Part model, mm, in its own coordinate system. Face numbers are marked on the shaded views. A direction names the side the tool comes from. Round coordinates to 2 decimals unless told otherwise and drop trailing zeros. Loops run counter-clockwise (first coordinate to the right, second up) from the corner with the lowest first, then second, coordinate; pieces in that order, holes last. Notation, with made-up numbers: (45, -30) - (90, -30) arc R17 cw to (90, -9) - close; hole circle Ø9 at (89.25, 32.25). An arc over 180 degrees is marked (long way). Write each question's results on one line, items separated by ' | '. Start each with the question number.
(1) Tool access for the marked faces 1, 2, 3, 4 and 5: list every direction of +Z, -Z, +X, -X, +Y, -Y with a clear straight run to the whole face (end or side of a thin tool).
(2) Cut at C-C, the plane y = 8. List the corners of the cut face in (x, z).
(3) Drill centre lines: L1, parallel to Z at x = 5.5, y = 2.2; L2, parallel to Z at x = 54.5, y = 22; L3, parallel to X at y = 1.45, z = -40.5. Where is each one in solid material? Low to high.
(4) Cut at A-A, the plane y = 29.5. List the corners of the cut face in (x, z), then the cut area to 3 significant figures.
(5) Flat gauge pins, fed straight in: P1, Ø11, axis at x = 53.5, z = -13, coming from the -Y side; P2, Ø8, axis at x = 35.5, y = 7.5, coming from the +Z side; P3, Ø5.5, axis at x = 52.5, z = -29.5, coming from the +Y side. Where does each tip first touch, or does it go through?
(6) Cut at B-B, the plane y = 17. List the corners of the cut face in (x, z), then the cut area to 3 significant figures.
(7) Cut at D-D, the plane z = 5. List the corners of the cut face in (x, y).
(8) Mould opens along Z. For the marked faces 6, 7, 8 and 9 say: released by +Z, released by -Z, zero draft, split by the parting line, or undercut.
from build123d import *

# Parameters (mm, degrees)
BOSS_EXTRUDE1_DEPTH = 3.8
SKETCH2_W           = 45.8
SKETCH2_H           = 50
BOSS_EXTRUDE2_DEPTH = 4
BOSS_EXTRUDE3_DEPTH = 46.2
BOSS_EXTRUDE4_DEPTH = 3.8
BOSS_EXTRUDE5_REACH = 52
SKETCH6_W           = 9
SKETCH6_H           = 50
BOSS_EXTRUDE6_DEPTH = 1
BOSS_EXTRUDE6_TAPER = 45
SKETCH7_R           = 2.6
BOSS_EXTRUDE7_DEPTH = 4
CUT_EXTRUDE1_REACH  = 6
SKETCH8_R           = 13
SKETCH8_R_2         = 1.6
SKETCH9_R           = 2.6
CUT_EXTRUDE2_DEPTH  = 4.8
SKETCH10_R          = 5
CUT_EXTRUDE3_DEPTH  = 20


with BuildPart() as part:
    # Sketch1 → Boss-Extrude1 (new body)
    with BuildSketch(Plane.XY):
        Polygon((0, 0), (45.8, 0), (64.164, 21.885362974), (64.164, 24.164), (44.164, 24.164), (44.164, 44.164), (40.164, 44.164), (0, 4), align=None)
    extrude(amount=-BOSS_EXTRUDE1_DEPTH)

    # Sketch2 → Boss-Extrude2 (add)
    with BuildSketch(Plane.XZ):
        with Locations((22.9, -25)):
            Rectangle(SKETCH2_W, SKETCH2_H)
    extrude(amount=-BOSS_EXTRUDE2_DEPTH)

    # Sketch3 → Boss-Extrude3 (add, through all)
    with BuildSketch(Plane(origin=(0, 0, -3.8), x_dir=(-1, 0, 0), z_dir=(0, 0, -1))):
        Polygon((-45.8, 0), (-45.8, 4), (-49.156398525, 4), align=None)
    extrude(amount=BOSS_EXTRUDE3_DEPTH)

    # Sketch4 → Boss-Extrude4 (add)
    with BuildSketch(Plane(origin=(0, 0, -50), x_dir=(-1, 0, 0), z_dir=(0, 0, -1))):
        Polygon((-44.164, 24.164), (-44.164, 44.164), (-40.164, 44.164), (0, 4), (0, 0), (-45.8, 0), (-64.164, 21.885362974), (-64.164, 24.164), align=None)
    extrude(amount=-BOSS_EXTRUDE4_DEPTH)

    # Sketch5 → Boss-Extrude5 (add, up to next)
    with BuildSketch(Plane.XY, mode=Mode.PRIVATE) as boss_extrude5_sk1:
        Polygon((44.164, 24.164), (44.164, 0), (45.8, 0), (64.164, 21.885362974), (64.164, 24.164), align=None)
    boss_extrude5_tool1 = extrude(boss_extrude5_sk1.sketch, amount=-BOSS_EXTRUDE5_REACH, mode=Mode.PRIVATE) - part.part
    add(boss_extrude5_tool1.solids().sort_by_distance((51.403304, 15.489129, 0))[0])

    # Sketch6 → Boss-Extrude6 (add)
    with BuildSketch(Plane(origin=(0, 24.164, 0), x_dir=(1, 0, 0), z_dir=(0, 1, 0))):
        with Locations((54.164, 25)):
            Rectangle(SKETCH6_W, SKETCH6_H)
    extrude(amount=BOSS_EXTRUDE6_DEPTH, taper=BOSS_EXTRUDE6_TAPER)

    # Sketch7 → Boss-Extrude7 (add)
    with BuildSketch(Plane(origin=(44.164, 0, 0), x_dir=(0, 0, -1), z_dir=(1, 0, 0))):
        with BuildLine():
            Line((0, 24.164), (0, 10.164))
            Line((0, 10.164), (-16.646029173, 27.168696786))
            ThreePointArc((-16.646029173, 27.168696786), (-18.718270774, 38.040013923), (-9.5, 44.164))
            Line((-9.5, 44.164), (3.8, 44.164))
            Line((3.8, 44.164), (3.8, 24.164))
            Line((3.8, 24.164), (0, 24.164))
        make_face()
        with Locations((-9.5, 34.164)):
            Circle(SKETCH7_R, mode=Mode.SUBTRACT)
        with BuildLine():
            Line((46.2, 44.164), (46.2, 24.164))
            Line((46.2, 24.164), (50, 24.164))
            Line((50, 24.164), (50, 10.164))
            Line((50, 10.164), (66.646029173, 27.168696786))
            ThreePointArc((66.646029173, 27.168696786), (68.718270774, 38.040013923), (59.5, 44.164))
            Line((59.5, 44.164), (46.2, 44.164))
        make_face()
        with Locations((59.5, 34.164)):
            Circle(SKETCH7_R, mode=Mode.SUBTRACT)
    extrude(amount=-BOSS_EXTRUDE7_DEPTH)

    # Sketch8 → Cut-Extrude1 (cut, up to next)
    with BuildSketch(Plane(origin=(0, 4, 0), x_dir=(1, 0, 0), z_dir=(0, 1, 0)), mode=Mode.PRIVATE) as cut_extrude1_sk1:
        with Locations((21, 25)):
            Circle(SKETCH8_R)
    cut_extrude1_tool1 = extrude(cut_extrude1_sk1.sketch, amount=-CUT_EXTRUDE1_REACH, mode=Mode.PRIVATE) & part.part
    add(cut_extrude1_tool1.solids().sort_by_distance((21, 4, -25))[0], mode=Mode.SUBTRACT)
    # Sketch8 → Cut-Extrude1 (cut, up to next)
    with BuildSketch(Plane(origin=(0, 4, 0), x_dir=(1, 0, 0), z_dir=(0, 1, 0)), mode=Mode.PRIVATE) as cut_extrude1_sk2:
        with Locations((5.5, 40.5)):
            Circle(SKETCH8_R_2)
    cut_extrude1_tool2 = extrude(cut_extrude1_sk2.sketch, amount=-CUT_EXTRUDE1_REACH, mode=Mode.PRIVATE) & part.part
    add(cut_extrude1_tool2.solids().sort_by_distance((5.5, 4, -40.5))[0], mode=Mode.SUBTRACT)
    # Sketch8 → Cut-Extrude1 (cut, up to next)
    with BuildSketch(Plane(origin=(0, 4, 0), x_dir=(1, 0, 0), z_dir=(0, 1, 0)), mode=Mode.PRIVATE) as cut_extrude1_sk3:
        with Locations((38.664, 40.5)):
            Circle(SKETCH8_R_2)
    cut_extrude1_tool3 = extrude(cut_extrude1_sk3.sketch, amount=-CUT_EXTRUDE1_REACH, mode=Mode.PRIVATE) & part.part
    add(cut_extrude1_tool3.solids().sort_by_distance((38.664, 4, -40.5))[0], mode=Mode.SUBTRACT)
    # Sketch8 → Cut-Extrude1 (cut, up to next)
    with BuildSketch(Plane(origin=(0, 4, 0), x_dir=(1, 0, 0), z_dir=(0, 1, 0)), mode=Mode.PRIVATE) as cut_extrude1_sk4:
        with Locations((38.664, 7.336)):
            Circle(SKETCH8_R_2)
    cut_extrude1_tool4 = extrude(cut_extrude1_sk4.sketch, amount=-CUT_EXTRUDE1_REACH, mode=Mode.PRIVATE) & part.part
    add(cut_extrude1_tool4.solids().sort_by_distance((38.664, 4, -7.336))[0], mode=Mode.SUBTRACT)
    # Sketch8 → Cut-Extrude1 (cut, up to next)
    with BuildSketch(Plane(origin=(0, 4, 0), x_dir=(1, 0, 0), z_dir=(0, 1, 0)), mode=Mode.PRIVATE) as cut_extrude1_sk5:
        with Locations((5.5, 7.336)):
            Circle(SKETCH8_R_2)
    cut_extrude1_tool5 = extrude(cut_extrude1_sk5.sketch, amount=-CUT_EXTRUDE1_REACH, mode=Mode.PRIVATE) & part.part
    add(cut_extrude1_tool5.solids().sort_by_distance((5.5, 4, -7.336))[0], mode=Mode.SUBTRACT)

    # Sketch9 → Cut-Extrude2 (cut)
    with BuildSketch(Plane(origin=(0, 25.164, 0), x_dir=(1, 0, 0), z_dir=(0, 1, 0))):
        with Locations((54.164, 14.5)):
            Circle(SKETCH9_R)
        with Locations((54.164, 35.5)):
            Circle(SKETCH9_R)
    extrude(amount=-CUT_EXTRUDE2_DEPTH, mode=Mode.SUBTRACT)

    # Sketch10 → Cut-Extrude3 (cut)
    with BuildSketch(Plane.XZ):
        with Locations((52, -14.5)):
            Circle(SKETCH10_R)
        with Locations((52, -35.5)):
            Circle(SKETCH10_R)
    extrude(amount=-CUT_EXTRUDE3_DEPTH, mode=Mode.SUBTRACT)


solid = part.part
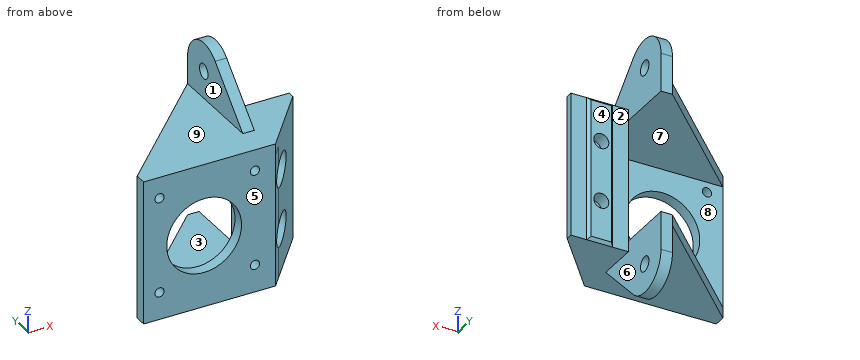
A:
1) face 1: +Z, -X, +Y, -Y | face 2: +Z, -Z, +Y | face 3: -X, +Y | face 4: +Z, -Z, +X, +Y | face 5: +Z, -Z, +X, -X, -Y
2) outline: (4, -50) - (52.51, -50) - (52.51, -40.47) arc R5 cw (long way) to (52.51, -30.53) - (52.51, -19.47) arc R5 cw (long way) to (52.51, -9.53) - (52.51, 0) - (4, 0) - (4, -3.8) - (44.16, -3.8) - (44.16, -46.2) - (4, -46.2) - close
3) L1: -50 to -42.1, -38.9 to -8.94, -5.74 to 0 | L2: -50 to -38.08, -32.92 to -17.08, -11.92 to 0 | L3: 0 to 3.9, 7.1 to 37.06, 40.26 to 47.02
4) outline: (25.5, -50) - (40.16, -50) - (40.16, -68.35) - (44.16, -68.35) - (44.16, -46.2) - (25.5, -46.2) - close; (25.5, -3.8) - (44.16, -3.8) - (44.16, 18.35) - (40.16, 18.35) - (40.16, 0) - (25.5, 0) - close | area: 289 mm2
5) P1: y = 3.03 | P2: z = 0 | P3: y = 25.16
6) outline: (13, -50) - (40.16, -50) - (40.16, -56.69) - (44.16, -56.69) - (44.16, -50) - (60.06, -50) - (60.06, 0) - (44.16, 0) - (44.16, 6.69) - (40.16, 6.69) - (40.16, 0) - (13, 0) - (13, -3.8) - (44.16, -3.8) - (44.16, -46.2) - (13, -46.2) - close; hole circle Ø10 at (52, -35.5); hole circle Ø10 at (52, -14.5) | area: 928 mm2
7) outline: (40.16, 15.27) - (44.16, 15.27) - (44.16, 44.16) - (40.16, 44.16) - close
8) face 6: zero draft | face 7: undercut | face 8: undercut | face 9: released by +Z
